Geometry: final body of the model. Coordinates: model frame, mm. Face numbers are marked on the shaded views. Coordinates: 2 decimals unless noted, no trailing zeros. Write each loop counter-clockwise with the first axis right and the second up, starting at its lowest first coordinate (ties: lowest second). Pieces come first, ordered by that corner, then holes. Notation, with made-up numbers: M 30,-29 L 78,-29 A17 cw 78,-18 Z; hole C -12,-31.5 d10. An arc over 180 degrees is marked long. Write item = value, one per line. Start each with the question number.
Item 1: Ray query, L1, parallel to Y at x = 0, z = 19.05; L2, parallel to Y at x = 0, z = 12; L3, parallel to X at y = -1.5, z = 7.5. Return the intervals inside material, ascending. Write a range as [from, to].
Item 2: Pull-direction query (X, two-part tool) for the marked faces 1 and 2; classes: +X half, -X half, draft (parallel to the pull), parting line (faces both ways), or undercut.
Item 3: Section C-C on z = 3.5. Output: boundary loops of the cut face in (x, y), plus the area to 3 significant figures.
Item 4: First-contact query: pin 1 Ø10 at (x, z) = (-0.5, 13.5) entering from -Y; pin 2 Ø4 at (x, z) = (5.5, 11.5) entering from +Y; pin 3 Ø8 at (y, z) = (3, 3) entering from +X; pin 4 Ø4 at (y, z) = (-6, 11) entering from +X. Flat tips, straight axial feed; report the tip coordinate or a pass-through.
Item 5: Section A-A on y = 0. Output: boundary loops of the cut face in (x, z) (1 decimal).
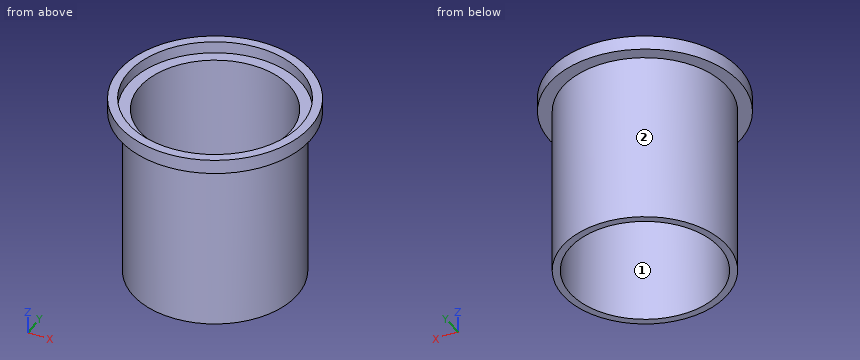
from build123d import *

# Parameters (mm, degrees)
F0_R     = 8.763
F1_DEPTH = 18.415
F3_R     = 10.16
F4_DEPTH = 1.524
F2_R     = 8.001
F5_DEPTH = 27.9654
F6_R     = 9.2075
F7_DEPTH = 1.27


with BuildPart() as f1:
    # F0 (on Top) → F1 (new body)
    with BuildSketch(Plane.XY):
        Circle(F0_R)
    extrude(amount=F1_DEPTH)

    # F3 (on face) → F4 (join)
    with BuildSketch(Plane.XY.offset(18.415)):
        Circle(F3_R)
    extrude(amount=F4_DEPTH)

    # F2 (on face) → F5 (cut, symmetric)
    with BuildSketch(Plane.XY.offset(18.415)):
        Circle(F2_R)
    extrude(amount=F5_DEPTH, both=True, mode=Mode.SUBTRACT)

    # F6 (on face) → F7 (cut)
    with BuildSketch(Plane.XY.offset(19.939)):
        Circle(F6_R)
    extrude(amount=-F7_DEPTH, mode=Mode.SUBTRACT)


solid = f1.part
Responses:
q1.L1 = [-10.16, -9.21], [9.21, 10.16]
q1.L2 = [-8.76, -8], [8, 8.76]
q1.L3 = [-8.63, -7.86], [7.86, 8.63]
q2.face_1 = undercut
q2.face_2 = parting line
q3.outline = C 0,0 d17.53; hole C 0,0 d16
q3.area = 40.1 mm²
q4.pin_1 = -10.16
q4.pin_2 = 8.03
q4.pin_3 = 8.76
q4.pin_4 = 7.8
q5.outline = M -10.2,18.4 L -8.8,18.4 L -8.8,0 L -8,0 L -8,18.7 L -9.2,18.7 L -9.2,19.9 L -10.2,19.9 Z; M 8,0 L 8.8,0 L 8.8,18.4 L 10.2,18.4 L 10.2,19.9 L 9.2,19.9 L 9.2,18.7 L 8,18.7 Z
